Could you check a few things on this model? Use its own coordinates, in mm. Face numbers are marked on the shaded views. Give positions to 0.01 mm unless a question says otherwise; leave off trailing zeros. Loops run counter-clockwise (first coordinate to the right, second up) from the corner with the lowest first, then second, coordinate; pieces in that order, holes last. Notation, with made-up numbers: (88, -15.75) -> (122, -15.75) arc R24 cw to (122, -5.75) -> close; hole circle Ø4 at (-21, 28.5). An arc over 180 degrees is marked (long way). Write each question's results on one line, items separated by ' | '. Start each with the question number.
Q1. Will these pins go through, and if not, where does the flat tip stop? P1, Ø0.8, axis at y = 54, z = -24, coming from the -X side; P2, Ø10, axis at y = 61, z = -17.5, coming from the +X side; P3, Ø4, axis at y = 3, z = -17, coming from the -X side; P4, Ø5, axis at x = 7.5, z = -19.5, coming from the -Y side.
Q2. If we section it at B-B, the plane z = -12.75: Give the number of separate pieces and of enclosed holes in the cut face, plus the area to 3 significant figures.
Q3. We'd pull the mould along X, two halves only. Please class the marked faces 1, 2 and 3: released by +X, released by -X, zero draft, split by the parting line, or undercut.
Q4. If I drill on line 1 along Y through (x, z) = (-33, -0.75); line 2 along Z through (x, y) = (13, 33.5); line 3 along X through (y, z) = (30.5, -5.25), over which ranges is the centre line in solid material (lowest first)?
Q5. If we section it at A-A, the plane x = -12: List the corners of the cut face in (y, z) for me.
from build123d import *

# Parameters (mm, degrees)
BOSS_EXTRUDE3_DEPTH                  = 95
FILLET8_R                            = 5
FILLET9_R                            = 5
FILLET10_R                           = 5
ESQUISSE3_W                          = 30
ESQUISSE3_H                          = 85
ENL_V_MAT_EXTRU_1_DEPTH              = 122.963109328
ESQUISSE5_W                          = 10
ESQUISSE5_H                          = 60
ENL_V_MAT_EXTRU_2_DEPTH              = 122.963109328
ESQUISSE14_W                         = 10
ESQUISSE14_H                         = 25
ENL_V_MAT_EXTRU_7_DEPTH              = 122.963109328
ESQUISSE15_W                         = 30
ESQUISSE15_H                         = 85
ENL_V_MAT_EXTRU_8_DEPTH              = 122.963109328
ESQUISSE21_W                         = 15
ESQUISSE21_H                         = 85
ENL_V_MAT_EXTRU_9_DEPTH              = 122.963109328
ESQUISSE61_W                         = 43.670119933
ESQUISSE61_H                         = 20.938302955
BOSS_EXTRU_3_DEPTH                   = 5
ENL_V_MAT_EXTRU_18_DEPTH             = 5
ESQUISSE69_W                         = 43.623857554
ESQUISSE69_H                         = 17.142891977
BOSS_EXTRU_4_DEPTH                   = 5
ENL_V_MAT_EXTRU_21_DEPTH             = 10
BOSS_EXTRU_7_DEPTH                   = 17
ENL_V_MAT_EXTRU_25_REACH             = 122.865
ENL_V_MAT_EXTRU_25_DIRECTION_2_DEPTH = 121.865309224
BOSS_EXTRU_10_DEPTH                  = 86
ESQUISSE84_R                         = 1
ENL_V_MAT_EXTRU_26_DEPTH             = 120.791485603


with BuildPart() as part:
    # Sketch1 → Boss-Extrude3 (new body)
    with BuildSketch(Plane(origin=(0, 0, 0), x_dir=(1, 0, 0), z_dir=(0, 1, 0))):
        Polygon((-75, 0), (-75, 10), (24.166666667, 10), (12.5, 20), (12.5, 25), (30, 10), (55.980762114, 25), (55.980762114, 20), (28.449754988, 3.036452995), (23.521740286, 0), align=None)
    extrude(amount=BOSS_EXTRUDE3_DEPTH)

    # Fillet8
    fillet8_edges = [part.edges().sort_by_distance(p)[0] for p in [
        (24.166666667, 47.5, -10),
    ]]
    fillet(fillet8_edges, radius=FILLET8_R)

    # Fillet9
    fillet9_edges = [part.edges().sort_by_distance(p)[0] for p in [
        (55.980762114, 47.5, -20),
        (12.5, 47.5, -20),
    ]]
    fillet(fillet9_edges, radius=FILLET9_R)

    # Fillet10
    fillet10_edges = [part.edges().sort_by_distance(p)[0] for p in [
        (23.521740286, 47.5, 0),
    ]]
    fillet(fillet10_edges, radius=FILLET10_R)

    # Esquisse3 → Enlèv. mat.-Extru.1 (cut, through all)
    with BuildSketch(Plane(origin=(0, 0, -10), x_dir=(-1, 0, 0), z_dir=(0, 0, -1))):
        with Locations((60, 47.5)):
            Rectangle(ESQUISSE3_W, ESQUISSE3_H)
    extrude(amount=-ENL_V_MAT_EXTRU_1_DEPTH, mode=Mode.SUBTRACT)

    # Esquisse5 → Enlèv. mat.-Extru.2 (cut, through all)
    with BuildSketch(Plane(origin=(0, 0, -10), x_dir=(-1, 0, 0), z_dir=(0, 0, -1))):
        with Locations((40, 35)):
            Rectangle(ESQUISSE5_W, ESQUISSE5_H)
    extrude(amount=-ENL_V_MAT_EXTRU_2_DEPTH, mode=Mode.SUBTRACT)

    # Esquisse14 → Enlèv. mat.-Extru.7 (cut, through all)
    with BuildSketch(Plane(origin=(0, 0, -10), x_dir=(-1, 0, 0), z_dir=(0, 0, -1))):
        with Locations((40, 77.5)):
            Rectangle(ESQUISSE14_W, ESQUISSE14_H)
    extrude(amount=-ENL_V_MAT_EXTRU_7_DEPTH, mode=Mode.SUBTRACT)

    # Esquisse15 → Enlèv. mat.-Extru.8 (cut, through all)
    with BuildSketch(Plane(origin=(0, 0, -10), x_dir=(-1, 0, 0), z_dir=(0, 0, -1))):
        with Locations((20, 47.5)):
            Rectangle(ESQUISSE15_W, ESQUISSE15_H)
    extrude(amount=-ENL_V_MAT_EXTRU_8_DEPTH, mode=Mode.SUBTRACT)

    # Esquisse21 → Enlèv. mat.-Extru.9 (cut, through all)
    with BuildSketch(Plane(origin=(0, 0, -10), x_dir=(-1, 0, 0), z_dir=(0, 0, -1))):
        with Locations((-2.5, 47.5)):
            Rectangle(ESQUISSE21_W, ESQUISSE21_H)
    extrude(amount=-ENL_V_MAT_EXTRU_9_DEPTH, mode=Mode.SUBTRACT)

    # Esquisse61 → Boss.-Extru.3 (add)
    with BuildSketch(Plane(origin=(0, 0, 0), x_dir=(1, 0, 0), z_dir=(0, 1, 0))):
        with Locations((34.105579197, 14.530848522)):
            Rectangle(ESQUISSE61_W, ESQUISSE61_H)
    extrude(amount=BOSS_EXTRU_3_DEPTH)

    # Esquisse63 → Enlèv. mat.-Extru.18 (cut)
    with BuildSketch(Plane(origin=(0, 5, 0), x_dir=(1, 0, 0), z_dir=(0, 1, 0))):
        Polygon((55.940639163, 22.159973494), (55.183036705, 20.082720902), (53.603647545, 18.535313491), (30.113675938, 4.061697045), (55.940639163, 4.061697045), align=None)
    extrude(amount=-ENL_V_MAT_EXTRU_18_DEPTH, mode=Mode.SUBTRACT)

    # Esquisse69 → Boss.-Extru.4 (add)
    with BuildSketch(Plane(origin=(0, 95, 0), x_dir=(1, 0, 0), z_dir=(0, 1, 0))):
        with Locations((34.168833337, 16.428554012)):
            Rectangle(ESQUISSE69_W, ESQUISSE69_H)
    extrude(amount=-BOSS_EXTRU_4_DEPTH)

    # Esquisse71 → Enlèv. mat.-Extru.21 (cut)
    with BuildSketch(Plane.XZ.offset(-90)):
        Polygon((55.980762114, -22.792128264), (55.826118619, -21.558223754), (55.346218971, -20.354345168), (54.812246486, -19.579694996), (53.603647545, -18.535313491), (36.273442327, -7.857108023), (55.980762114, -7.857108023), align=None)
    extrude(amount=-ENL_V_MAT_EXTRU_21_DEPTH, mode=Mode.SUBTRACT)

    # Esquisse77 → Boss.-Extru.7 (add)
    with BuildSketch(Plane(origin=(3.169872981, 0, 5.490381057), x_dir=(-0.8660254037844384, 0, 0.5000000000000004), z_dir=(-0.5000000000000004, 0, -0.8660254037844384))):
        Polygon((-30.980762114, 90), (-40.980762114, 90), (-31.480762114, 5), (-30.980762114, 5), align=None)
    extrude(amount=BOSS_EXTRU_7_DEPTH)

    # Esquisse79 → Enlèv. mat.-Extru.25 (cut, up to next)
    with BuildSketch(Plane(origin=(0, 90, 0), x_dir=(1, 0, 0), z_dir=(0, 1, 0)), mode=Mode.PRIVATE) as enl_v_mat_extru_25_sk1:
        Polygon((21.980762114, 25), (32.886751346, 25), (30.160254038, 29.722431864), align=None)
    enl_v_mat_extru_25_tool1 = extrude(enl_v_mat_extru_25_sk1.sketch, amount=-ENL_V_MAT_EXTRU_25_REACH, mode=Mode.PRIVATE) & part.part
    add(enl_v_mat_extru_25_tool1.solids().sort_by_distance((28.342589, 90, -26.574144))[0], mode=Mode.SUBTRACT)

    # Esquisse79 → Enlèv. mat.-Extru.25 direction 2 (cut)
    with BuildSketch(Plane(origin=(0, 90, 0), x_dir=(1, 0, 0), z_dir=(0, 1, 0))):
        Polygon((21.980762114, 25), (32.886751346, 25), (30.160254038, 29.722431864), align=None)
    extrude(amount=ENL_V_MAT_EXTRU_25_DIRECTION_2_DEPTH, mode=Mode.SUBTRACT)

    # Esquisse80 → Boss.-Extru.10 (add)
    with BuildSketch(Plane(origin=(0, 5, 0), x_dir=(1, 0, 0), z_dir=(0, 1, 0))):
        Polygon((12.5, 25), (30, 10), (21.25, 25), align=None)
    extrude(amount=BOSS_EXTRU_10_DEPTH)

    # Esquisse84 → Enlèv. mat.-Extru.26 (cut, through all)
    with BuildSketch(Plane(origin=(0, 90, 0), x_dir=(-1, 0, 0), z_dir=(0, -1, 0))):
        with Locations(Location((70, 5, 0), (0, 0, 90))):
            Circle(ESQUISSE84_R)
        with Locations(Location((67, 5, 0), (0, 0, 90))):
            Circle(ESQUISSE84_R)
        with Locations(Location((64, 5, 0), (0, 0, 90))):
            Circle(ESQUISSE84_R)
        with Locations(Location((61, 5, 0), (0, 0, 90))):
            Circle(ESQUISSE84_R)
        with Locations(Location((41, 5, 0), (0, 0, 90))):
            Circle(ESQUISSE84_R)
        with Locations(Location((38, 5, 0), (0, 0, 90))):
            Circle(ESQUISSE84_R)
        with Locations(Location((35, 5, 0), (0, 0, 90))):
            Circle(ESQUISSE84_R)
        with Locations(Location((32, 5, 0), (0, 0, 90))):
            Circle(ESQUISSE84_R)
    extrude(amount=-ENL_V_MAT_EXTRU_26_DEPTH, mode=Mode.SUBTRACT)


solid = part.part
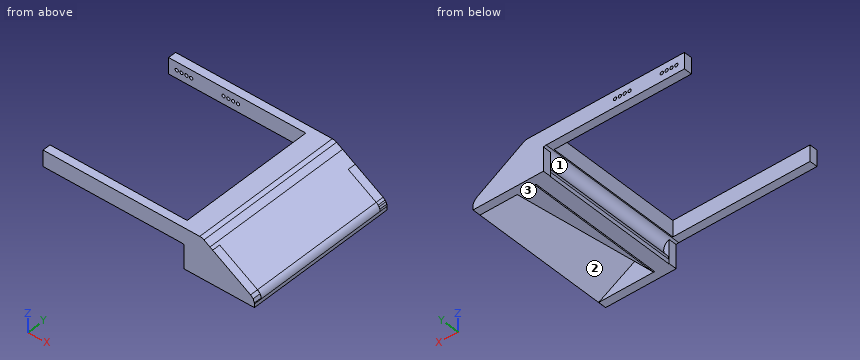
Final values:
1) P1: stops at x = 12.5 | P2: stops at x = 55.97 | P3: stops at x = 12.27 | P4: passes through
2) separate pieces: 1 | enclosed holes: 2 | area: 2,660 mm²
3) face 1: released by -X | face 2: undercut | face 3: zero draft
4) line 1: y = 0 to 5, 90 to 95 | line 2: z = -25 to -20.11, -10.59 to 0 | line 3: x = 10 to 32.04
5) outline: (0, -10) -> (5, -10) -> (5, 0) -> (0, 0) -> close; (90, -10) -> (95, -10) -> (95, 0) -> (90, 0) -> close
